The figure shows three views and two pictorial views of one solid part (mm, origin at its lowest corner). Answer the questions. A direction names the side the tool comes from. Coordinates: 2 decimals unless noted, no trailing zeros. Order: outer loops, then holes, each group sorted by start corner. A loop starts at its lowest first (then second) coordinate and runs counter-clockwise, first axis right, second up. Notation, with made-up numbers: (62.5, 32.5) -> (108.5, 32.5) arc R35 cw to (108.5, 71.5) -> close; hole circle Ø5 at (63.5, -2.5). An arc over 180 degrees is marked (long way). Write item = value, one per line.
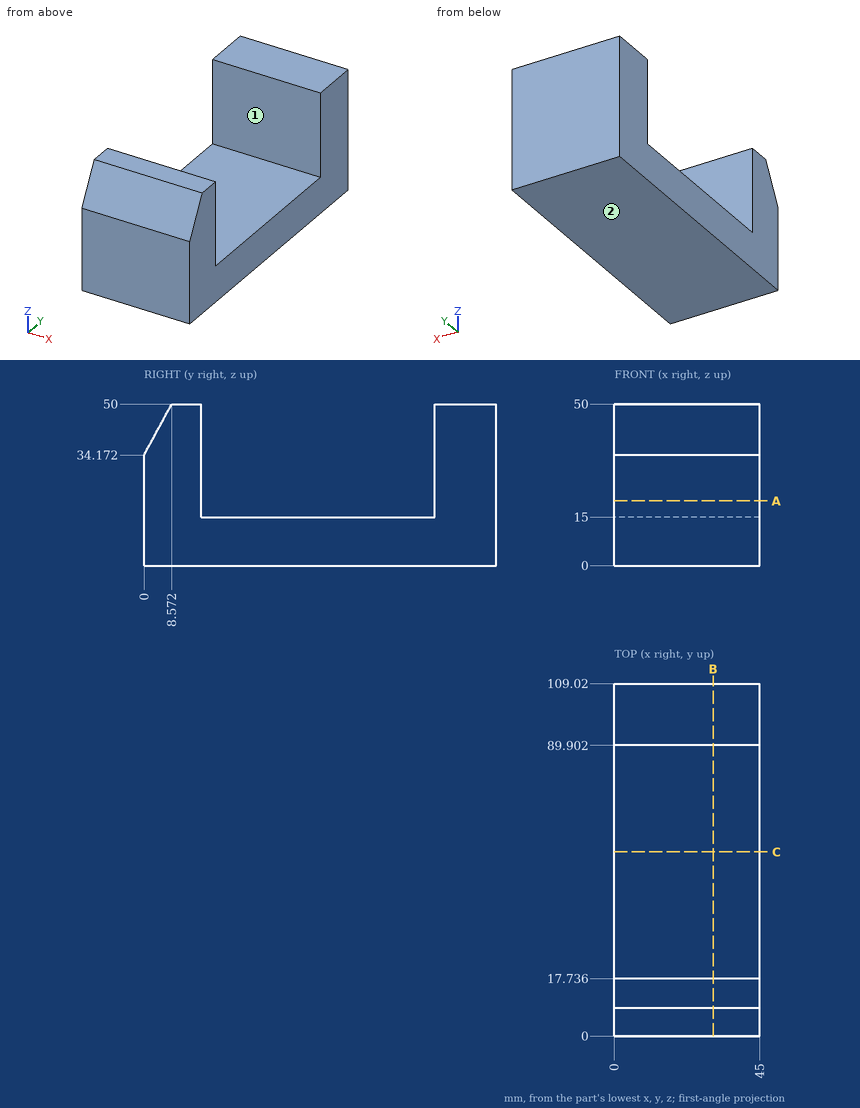
Q1. Section C-C, the plane y = 57 is taken. Give the vertices of the cut face in (x, z).
The answers:
outline = (0, 0) -> (45, 0) -> (45, 15) -> (0, 15) -> close
Q2. Find the intervals of material crossed by line 1 along Y through (x, z) = (20, 16.5); line 2 along Z through (x, y) = (34, 59); line 3 along Y through (x, z) = (32, 41) (1 decimal), in increasing order.
The answers:
line_1 = 0 to 17.74, 89.9 to 109.02
line_2 = 0 to 15
line_3 = 3.7 to 17.7, 89.9 to 109
Q3. Section A-A, the plane z = 20 is taken. Give the vertices of the cut face in (x, y), plus the area to 3 significant figures.
The answers:
outline = (0, 0) -> (45, 0) -> (45, 17.74) -> (0, 17.74) -> close; (0, 89.9) -> (45, 89.9) -> (45, 109.02) -> (0, 109.02) -> close
area = 1,660 mm2
Q4. A tool of negligible diameter and unlimited length cuts with its end or side. For the marked faces 1 and 2, from which of +Z, -Z, +X, -X, +Y, -Y can it reach the whole face along a straight path? Write none if from no direction.
The answers:
face_1 = +Z, +X, -X
face_2 = -Z, +X, -X, +Y, -Y
Q5. This flat-tipped pin is pushed along its axis until it touches: pin 1 Ø12 at (x, y) = (6.5, 60) entering from +Z. Where does it stop, or does it pass through?
The answers:
pin_1 = 15
Q6. Section B-B, the plane x = 30.5 is taken. Give the vertices of the cut face in (y, z), plus the area to 3 significant figures.
The answers:
outline = (0, 0) -> (109.02, 0) -> (109.02, 50) -> (89.9, 50) -> (89.9, 15) -> (17.74, 15) -> (17.74, 50) -> (8.57, 50) -> (0, 34.17) -> close
area = 2,860 mm2
